Source: CAD feature listing. Evaluate the final solid. Frame: model axes, mm. Give positions to 0.01 mm unless a question says otherwise; leave off trailing zeros. Order: outer loops, then holes, each group sorted by start corner. A loop starts at its lowest first (then second) coordinate and runs counter-clockwise, first axis right, second up.
1) First-contact query: P1, Ø8, axis at y = 16, z = 9, coming from the -X side. Flat tip, straight axial feed; report the tip coordinate or a pass-through.
2) Section C-C, the plane y = 10.75. Return loops of the section in (x, z), plus the area to 3 significant figures.
3) Section A-A, the plane z = 11.25. Return loops of the section in (x, y).
4) Section B-B, the plane x = 10.5. Return loops of the section in (y, z).
5) Material intervals for line 1 (Y direction, x = 10, z = 17.75); line 2 (X direction, y = 9, z = 19); line 3 (X direction, y = 10.75, z = 9.5), sorted ascending.
```python
from build123d import *

# Parameters (mm, degrees)
F1_DEPTH = 20


with BuildPart() as f1:
    # F0 (on Top) → F1 (new body)
    with BuildSketch(Plane.XY):
        with BuildLine():
            Line((0, 10), (0, 0))
            Line((0, 0), (10, 0))
            Line((10, 0), (10, 8.5))
            ThreePointArc((10, 8.5), (8.93934, 8.93934), (8.5, 10))
            Line((8.5, 10), (0, 10))
        make_face()
        with BuildLine():
            Line((10, 8.5), (10, 0))
            Line((10, 0), (20, 0))
            Line((20, 0), (20, 10))
            Line((20, 10), (11.5, 10))
            ThreePointArc((11.5, 10), (11.06066, 8.93934), (10, 8.5))
        make_face()
        with BuildLine():
            Line((0, 20), (0, 10))
            Line((0, 10), (8.5, 10))
            ThreePointArc((8.5, 10), (8.93934, 11.06066), (10, 11.5))
            Line((10, 11.5), (10, 20))
            Line((10, 20), (0, 20))
        make_face()
        with BuildLine():
            Line((11.5, 10), (20, 10))
            Line((20, 10), (20, 20))
            Line((20, 20), (10, 20))
            Line((10, 20), (10, 11.5))
            ThreePointArc((10, 11.5), (11.06066, 11.06066), (11.5, 10))
        make_face()
    extrude(amount=F1_DEPTH)


solid = f1.part
```
From the geometry:
1. P1: stops at x = 0
2. outline: (0, 0) - (8.7, 0) - (8.7, 20) - (0, 20) - close; (11.3, 0) - (20, 0) - (20, 20) - (11.3, 20) - close
2. area: 348 mm2
3. outline: (0, 0) - (20, 0) - (20, 20) - (0, 20) - close; hole (8.5, 10) arc R1.5 ccw to (10, 8.5) arc R1.5 ccw to (11.5, 10) arc R1.5 ccw to (10, 11.5) arc R1.5 ccw to start
4. outline: (0, 0) - (8.59, 0) - (8.59, 20) - (0, 20) - close; (11.41, 0) - (20, 0) - (20, 20) - (11.41, 20) - close
5. line 1: y = 0 to 8.5, 11.5 to 20
5. line 2: x = 0 to 8.88, 11.12 to 20
5. line 3: x = 0 to 8.7, 11.3 to 20
